Geometry check sheet. Reference: the model listing, model coordinates, mm. A direction names the side the tool comes from. Round coordinates to 2 decimals unless told otherwise and drop trailing zeros. Loops run counter-clockwise (first coordinate to the right, second up) from the corner with the lowest first, then second, coordinate; pieces in that order, holes last.
Autodesk Fusion 360 part; units mm, degrees
sketch "Sketch1" plane through (0, 0, 0) normal (0, 0, 1) x (1, 0, 0)
  line L0 (2, 0) -> (162, 0)
  line L1 (164, 2) -> (164, 172)
  line L2 (162, 174) -> (2, 174)
  line L3 (0, 172) -> (0, 2)
  arc A0 (2, 174) -> (0, 172) centre (2, 172) ccw
  arc A1 (164, 172) -> (162, 174) centre (162, 172) ccw
  arc A2 (0, 2) -> (2, 0) centre (2, 2) ccw
  arc A3 (162, 0) -> (164, 2) centre (162, 2) ccw
  point P0 (164, 0)
  point P1 (0, 174)
  dimension "d1" = 164
  dimension "d2" = 174
  dimension "d3" = 2
  dimension "d4" = 2
  dimension "d5" = 2
  dimension "d6" = 2
extrude "Extrude1" add sketch "Sketch1" along normal blind 14
sketch "Sketch4" plane through (0, 0, 14) normal (0, 0, 1) x (-1, 0, 0)
  arc A0 (-162, 0) -> (-164, -2) centre (-162, -2) ccw
  line L0 (-164, -2) -> (-164, -172)
  arc A1 (-164, -172) -> (-162, -174) centre (-162, -172) ccw
  line L1 (-162, -174) -> (-2, -174)
  arc A2 (-2, -174) -> (0, -172) centre (-2, -172) ccw
  line L2 (0, -172) -> (0, -2)
  arc A3 (0, -2) -> (-2, 0) centre (-2, -2) ccw
  line L3 (-2, 0) -> (-162, 0)
  line L4 (-1.1, -172.9) -> (-162.9, -172.9)
  line L5 (-162.9, -172.9) -> (-162.9, -1.1)
  line L6 (-162.9, -1.1) -> (-1.1, -1.1)
  line L7 (-1.1, -1.1) -> (-1.1, -172.9)
  dimension "d19" = 161.8
  dimension "d20" = 171.8
  dimension "d21" = 1.1
  dimension "d22" = 1.1
extrude "Extrude4" add sketch "Sketch4" along normal blind 5 contours L4 L5 L6 L7
sketch "Sketch5" plane through (0, 0, 19) normal (0, 0, 1) x (-1, 0, 0)
  line L0 (-1.1, -1.1) -> (-162.9, -1.1)
  line L1 (-162.9, -1.1) -> (-162.9, -172.9)
  line L2 (-162.9, -172.9) -> (-1.1, -172.9)
  line L3 (-1.1, -172.9) -> (-1.1, -1.1)
  line L4 (-1.9, -172.1) -> (-162.1, -172.1)
  line L5 (-162.1, -172.1) -> (-162.1, -1.9)
  line L6 (-162.1, -1.9) -> (-1.9, -1.9)
  line L7 (-1.9, -1.9) -> (-1.9, -172.1)
  dimension "d25" = 160.2
  dimension "d26" = 170.2
  dimension "d27" = 0.8
  dimension "d28" = 0.8
extrude "Extrude5" cut sketch "Sketch5" against normal blind 5 contours L4 L5 L6 L7
sketch "Sketch6" plane through (0, 0, 14) normal (0, 0, 1) x (-1, 0, 0)
  line L0 (-1.9, -1.9) -> (-162.1, -1.9)
  line L1 (-162.1, -1.9) -> (-162.1, -172.1)
  line L2 (-162.1, -172.1) -> (-1.9, -172.1)
  line L3 (-1.9, -172.1) -> (-1.9, -1.9)
  line L4 (-2.9, -171.1) -> (-160.9, -171.1)
  line L5 (-160.9, -171.1) -> (-160.9, -3.1)
  line L6 (-160.9, -3.1) -> (-2.9, -3.1)
  line L7 (-2.9, -3.1) -> (-2.9, -171.1)
  dimension "d31" = 158
  dimension "d32" = 168
  dimension "d33" = 1
  dimension "d34" = 1
extrude "Extrude6" cut sketch "Sketch6" against normal blind 11.5 contours L4 L5 L6 L7
sketch "Sketch9" plane through (0, 0, 2.5) normal (0, 0, 1) x (-1, 0, 0)
  line L0 (-2.9, -3.1) -> (-160.9, -3.1)
  line L1 (-160.9, -3.1) -> (-160.9, -171.1)
  line L2 (-160.9, -171.1) -> (-2.9, -171.1)
  line L3 (-2.9, -171.1) -> (-2.9, -3.1)
  line L4 (-10.9, -16.1) -> (-147.9, -16.1)
  line L5 (-147.9, -16.1) -> (-147.9, -36.1)
  line L6 (-147.9, -36.1) -> (-10.9, -36.1)
  line L7 (-10.9, -36.1) -> (-10.9, -16.1)
  dimension "d37" = 137
  dimension "d38" = 20
  dimension "d39" = 13
  dimension "d40" = 8
extrude "Extrude7" cut sketch "Sketch9" against normal blind 2.5 contours L4 L5 L6 L7
sketch "Sketch10" plane through (0, 0, 0) normal (0, -1, 0) x (1, 0, 0)
  line L0 (2, 0) -> (162, 0)
  line L1 (162, 0) -> (162, 14)
  line L2 (162, 14) -> (2, 14)
  line L3 (2, 14) -> (2, 0)
  line L4 (66, 10) -> (72, 10)
  line L5 (72, 10) -> (72, 4)
  line L6 (72, 4) -> (66, 4)
  line L7 (66, 4) -> (66, 10)
  dimension "d43" = 6
  dimension "d44" = 6
  dimension "d45" = 4
  dimension "d46" = 64
sketch "Sketch11" plane through (0, 0, 0) normal (0, -1, 0) x (1, 0, 0)
  line L0 (92, 10) -> (98, 10)
  line L1 (98, 10) -> (98, 4)
  line L2 (98, 4) -> (92, 4)
  line L3 (92, 4) -> (92, 10)
  line L4 (162, 14) -> (2, 14)
  line L5 (162, 0) -> (162, 14)
  dimension "d47" = 6
  dimension "d48" = 6
  dimension "d49" = 4
  dimension "d50" = 64
extrude "Extrude8" cut sketch "Sketch10" against normal blind 3 contours L4 L5 L6 L7
extrude "Extrude9" cut sketch "Sketch11" against normal blind 3
sketch "Sketch12" plane through (0, 174, 0) normal (0, 1, 0) x (-1, 0, 0)
  line L0 (-162, 0) -> (-2, 0)
  line L1 (-2, 0) -> (-2, 14)
  line L2 (-2, 14) -> (-162, 14)
  line L3 (-162, 14) -> (-162, 0)
  line L4 (-142, 11) -> (-130, 11)
  line L5 (-130, 11) -> (-130, 3)
  line L6 (-130, 3) -> (-142, 3)
  line L7 (-142, 3) -> (-142, 11)
  dimension "d55" = 12
  dimension "d56" = 8
  dimension "d57" = 20
  dimension "d58" = 3
sketch "Sketch13" plane through (0, 174, 0) normal (0, 1, 0) x (-1, 0, 0)
  circle A0 centre (-110, 7) radius 1.5
  line L0 (-130, 11) -> (-130, 3)
  line L1 (-2, 14) -> (-162, 14)
  dimension "d59" = 3
  dimension "d60" = 20
  dimension "d61" = 7
extrude "Extrude10" cut sketch "Sketch12" against normal blind 3 contours L4 L5 L6 L7
extrude "Extrude11" cut sketch "Sketch13" against normal blind 3
fillet "Fillet1" radius 2 8 edges at (82, 174, 0) (0.5858, 173.4142, 0) (0, 87, 0) (0.5858, 0.5858, 0) (82, 0, 0) (163.4142, 0.5858, 0) (164, 87, 0) (163.4142, 173.4142, 0)
1) Sectioned sample at A-A, the plane y = 25.5. Record the cut outline in (x, z).
Report:
outline: (0, 2) arc R2 ccw to (2, 0) - (10.9, 0) - (10.9, 2.5) - (2.9, 2.5) - (2.9, 14) - (1.9, 14) - (1.9, 19) - (1.1, 19) - (1.1, 14) - (0, 14) - close; (147.9, 0) - (162, 0) arc R2 ccw to (164, 2) - (164, 14) - (162.9, 14) - (162.9, 19) - (162.1, 19) - (162.1, 14) - (160.9, 14) - (160.9, 2.5) - (147.9, 2.5) - close
2) Access from +Z, -Z, +X, -X, +Y, -Y to the whole of each face (thin tool, end or side, straight path). Record for faces 1 (the face through (81, 171.1, 8)), 2 (the face through (81, 172.9, 16)), 3 (the face through (83, 1.1, 16)).
Report:
face 1: +Z
face 2: +Z, +X, -X, +Y
face 3: +Z, +X, -X, -Y
3) Scan lines: line 1 along Y through (x, z) = (147.5, 16); line 2 along X through (y, z) = (128.5, 14.5); line 3 along Y through (x, z) = (91, 13.5). Record each from-to range of solid material in increasing order.
Report:
line 1: y = 1.1 to 1.9, 172.1 to 172.9
line 2: x = 1.1 to 1.9, 162.1 to 162.9
line 3: y = 0 to 3.1, 171.1 to 174
4) Gauge pin test, flat ends, axial feed: pin 1 (1.8 mm diameter, centred on x = 93.5, z = 5.5, fed in from -Y); pin 2 (4 mm diameter, centred on y = 99.5, z = 16.5, fed in from -X); pin 3 (0.8 mm diameter, centred on x = 101.5, z = 1, fed in from -Y). Record the tip position at first contact, or that the pin passes through.
Report:
pin 1: stops at y = 3
pin 2: stops at x = 1.1
pin 3: stops at y = 0.09
5) Sectioned sample at B-B, the plane x = 42.5. Record the cut outline in (y, z).
Report:
outline: (0, 2) arc R2 ccw to (2, 0) - (16.1, 0) - (16.1, 2.5) - (3.1, 2.5) - (3.1, 14) - (1.9, 14) - (1.9, 19) - (1.1, 19) - (1.1, 14) - (0, 14) - close; (36.1, 0) - (172, 0) arc R2 ccw to (174, 2) - (174, 14) - (172.9, 14) - (172.9, 19) - (172.1, 19) - (172.1, 14) - (171.1, 14) - (171.1, 2.5) - (36.1, 2.5) - close
6) Sectioned sample at C-C, the plane y = 76.5. Record the cut outline in (x, z).
Report:
outline: (0, 2) arc R2 ccw to (2, 0) - (162, 0) arc R2 ccw to (164, 2) - (164, 14) - (162.9, 14) - (162.9, 19) - (162.1, 19) - (162.1, 14) - (160.9, 14) - (160.9, 2.5) - (2.9, 2.5) - (2.9, 14) - (1.9, 14) - (1.9, 19) - (1.1, 19) - (1.1, 14) - (0, 14) - close
